The model under review builds one solid part; all positions refer to its coordinate system, in mm. A direction names the side the tool comes from. Round coordinates to 2 decimals unless told otherwise and drop trailing zeros. Write each loop counter-clockwise with the first axis right and the second up, starting at its lowest first coordinate (ties: lowest second). Pieces come first, ordered by that corner, then holes. Notation, with made-up numbers: (28.25, -9) -> (45.25, -9) arc R18 cw to (45.25, 21) -> close; hole circle Ø4 at (65.25, 56.25). An arc over 180 degrees is marked (long way). Use CSV: the item, a comma, the result in double quotes. Start each with the question number.
1) Machinability: for faces 1 (the face through (1.588, 343, 2)), 2 (the face through (0, 350, 0)), which of the approach directions +Z, -Z, +X, -X, +Y, -Y give a long, thin tool a straight path to every point of the face, cutting with its end or side? Answer none if there is none.
2) Take a section at D-D, the plane y = 344.5. Give the boundary of the cut face in (x, z) (1 decimal), then the cut area to 3 significant figures.
3) Take a section at A-A, the plane y = 341.25. Give the boundary of the cut face in (x, z) (1 decimal), then the cut area to 3 significant figures.
4) Mouldability with a two-part tool opening along X and no side actions: class faces 3 (the face through (0, 350, 3.175)), 4 (the face through (-1.588, 343, 2)), 5 (the face through (-14.352, 346.379, 1.61)) as released by +X, released by -X, zero draft, split by the parting line, or undercut.
5) For pin 1 Ø1 at (x, z) = (0.5, 2) entering from -Y (3 decimals); pin 2 Ø1.6 at (y, z) = (343.5, 1) entering from -X; pin 3 Ø1.6 at (y, z) = (345, 1) entering from +X, all flat-tipped, find the tip position at first contact; note any pin that passes through.
6) Take a section at C-C, the plane x = 21. Give the boundary of the cut face in (y, z) (3 decimals).
7) Wall thickness on probe 1 along X at (y, z) = (347.5, 2.4); probe 2 along X at (y, z) = (340.25, 0.95); probe 3 along X at (y, z) = (354.25, 2.95): over which ranges is each line inside the solid? List them lowest first. Write a range as [from, to].
8) Take a section at B-B, the plane z = 1.3. Give the boundary of the cut face in (x, y), then the cut area to 3 significant figures.
from build123d import *

# Parameters (mm, degrees)
BOSS_EXTRUDE1_DEPTH = 1.5875


with BuildPart() as part:
    # Sketch2 → Boss-Extrude1 (new, symmetric)
    with BuildSketch(Plane.XY.offset(1.5875)):
        with BuildLine():
            ThreePointArc((-25, 356.408412891), (-14.187505021, 346.252036042), (-1.5875, 338.422482296))
            Line((-1.5875, 338.422482296), (-1.5875, 347.664977579))
            ThreePointArc((-1.5875, 347.664977579), (0, 349.252477579), (1.5875, 347.664977579))
            Line((1.5875, 347.664977579), (1.5875, 338.422482296))
            ThreePointArc((1.5875, 338.422482296), (14.187505021, 346.252036042), (25, 356.408412891))
            ThreePointArc((25, 356.408412891), (0, 357.65994376), (-25, 356.408412891))
        make_face()
        with BuildLine():
            Line((-1.5875, 347.664977579), (1.5875, 347.664977579))
            ThreePointArc((1.5875, 347.664977579), (0, 349.252477579), (-1.5875, 347.664977579))
        make_face()
    extrude(amount=BOSS_EXTRUDE1_DEPTH, both=True)


solid = part.part
Values found:
1,face 1,"+Z, -Z, -Y"
1,face 2,"-Z, +X, -X, +Y, -Y"
2,outline,"(-11.8, 0) -> (-1.6, 0) -> (-1.6, 3.2) -> (-11.8, 3.2) -> close; (1.6, 0) -> (11.8, 0) -> (11.8, 3.2) -> (1.6, 3.2) -> close"
2,area,"64.9 mm²"
3,outline,"(-6.8, 0) -> (-1.6, 0) -> (-1.6, 3.2) -> (-6.8, 3.2) -> close; (1.6, 0) -> (6.8, 0) -> (6.8, 3.2) -> (1.6, 3.2) -> close"
3,area,"33.1 mm²"
4,face 3,"zero draft"
4,face 4,"undercut"
4,face 5,"released by -X"
5,pin 1,"y = 347.665"
5,pin 2,"x = -11.53"
5,pin 3,"x = 13.59"
6,outline,"(352.17, 0) -> (356.778, 0) -> (356.778, 3.175) -> (352.17, 3.175) -> close"
7,probe 1,"[-15.77, -1.59], [1.59, 15.77]"
7,probe 2,"[-5.07, -1.59], [1.59, 5.07]"
7,probe 3,"[-23.04, 23.04]"
8,outline,"(-25, 356.41) arc R75 ccw to (-1.59, 338.42) -> (-1.59, 347.66) -> (1.59, 347.66) -> (1.59, 338.42) arc R75 ccw to (25, 356.41) arc R250.32 ccw to start"
8,area,"548 mm²"
